from build123d import *

# Parameters (mm, degrees)
F0_W     = 70
F0_H     = 40
F1_DEPTH = 30
F2_T     = -3
F3_W     = 34
F3_H     = 1
F4_DEPTH = 67


with BuildPart() as f1:
    # F0 (on Top) → F1 (new body)
    with BuildSketch(Plane.XY):
        Rectangle(F0_W, F0_H)
    extrude(amount=F1_DEPTH)

    # F2
    f2_openings = [f1.faces().sort_by_distance(p)[0] for p in [
        (0, 0, 30),
    ]]
    offset(amount=F2_T, openings=f2_openings)

    # F3 (on face) → F4 (cut, through all)
    with BuildSketch(Plane(origin=(-35, 0, 0), x_dir=(0, -1, 0), z_dir=(-1, 0, 0))):
        Polygon((-18.5, 27.5), (-18.5, 27), (18.5, 27), (18.5, 27.5), (17, 29), (-17, 29), align=None)
        with Locations((0, 29.5)):
            Rectangle(F3_W, F3_H)
    extrude(amount=-F4_DEPTH, mode=Mode.SUBTRACT)


solid = f1.part
The listing builds one solid part. Answer for the finished solid, in the listing's coordinates (mm). A direction names the side the tool comes from. Give positions to 0.01 mm unless a question says otherwise; leave off trailing zeros. Write each loop counter-clockwise with the first axis right and the second up, starting at its lowest first coordinate (ties: lowest second). Pieces come first, ordered by that corner, then holes.
1) Given P1, Ø18.5, axis at x = 4.5, y = 3.5, coming from the +Z side, flat-ended and moving along its own axis, determine where the tip first touches the part or whether it passes through.
2) Section B-B (y = -15.5) is taken. Write down the section's boundary in (x, z), and give its area (3 significant figures).
3) For a pull along Z with two mould halves and no side action, classify faces 1 (the face through (0, 0, 0)), 2 (the face through (-12, 18, 27)), 3 (the face through (0, 20, 15)) as pulls with the +Z half, pulls with the -Z half, needs draft (parallel to the pull), parting line crosses it, or undercut.
4) Find the intervals of material crossed by L1, parallel to Y at x = -26, z = 13.5; L2, parallel to X at y = -5.5, z = 21.75; L3, parallel to Y at x = -21.5, z = 27.5, in increasing order.
5) A tool of negligible diameter and unlimited length cuts with its end or side. For faces 4 (the face through (-2, 18, 28)), 5 (the face through (5, -18, 30)), 6 (the face through (0, 17, 15)), from which of +Z, -Z, +X, -X, +Y, -Y can it reach the whole face along a straight path? Write none if from no direction.
6) Section C-C (x = 4.5) is taken. Write down the section's boundary in (y, z).
7) Section A-A (z = 20.75) is taken. Write down the section's boundary in (x, y), and give its area (3 significant figures).
Response:
1. P1: stops at z = 3
2. outline: (-35, 0) - (35, 0) - (35, 30) - (32, 30) - (32, 3) - (-32, 3) - (-32, 27) - (-35, 27) - close
2. area: 363 mm2
3. face 1: pulls with the -Z half
3. face 2: undercut
3. face 3: needs draft
4. L1: y = -20 to -17, 17 to 20
4. L2: x = -35 to -32, 32 to 35
4. L3: y = -20 to -18.5, 18.5 to 20
5. face 4: -X
5. face 5: +Z, +X, -X, +Y, -Y
5. face 6: +Z
6. outline: (-20, 0) - (20, 0) - (20, 30) - (17, 30) - (17, 29) - (18.5, 27.5) - (18.5, 27) - (17, 27) - (17, 3) - (-17, 3) - (-17, 27) - (-18.5, 27) - (-18.5, 27.5) - (-17, 29) - (-17, 30) - (-20, 30) - close
7. outline: (-35, -20) - (35, -20) - (35, 20) - (-35, 20) - close; hole (-32, -17) - (32, -17) - (32, 17) - (-32, 17) - close
7. area: 624 mm2
